Could you check a few things on this model? Use its own coordinates, in mm. Round coordinates to 2 decimals unless told otherwise and drop trailing zeros. Loops run counter-clockwise (first coordinate to the right, second up) from the corner with the lowest first, then second, coordinate; pieces in that order, holes last. Notation, with made-up numbers: (58, -14.5) -> (110, -14.5) arc R36 cw to (110, 23.5) -> close; hole circle Ø3 at (-4, -13.5). An arc over 180 degrees is marked (long way). Write each question's results on one line, items separated by ' | '.
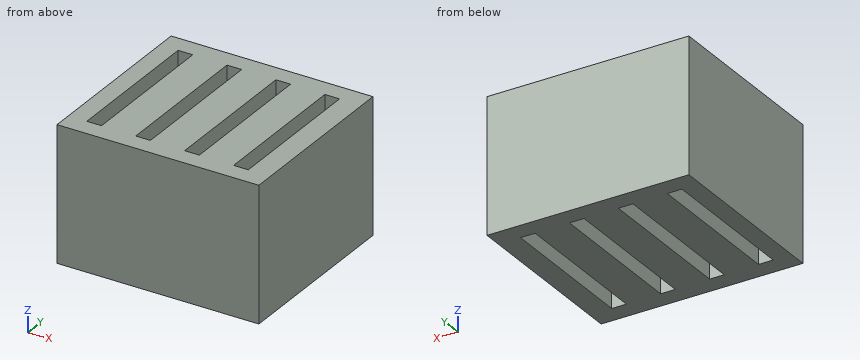
from build123d import *

# Parameters (mm, degrees)
BOX004_W     = 2.4
BOX004_H     = 24
BOX004_DEPTH = 22
BOX002_W     = 2.4
BOX002_H     = 24
BOX002_DEPTH = 22
BOX001_W     = 2.4
BOX001_H     = 24
BOX001_DEPTH = 22
BOX003_W     = 2.4
BOX003_H     = 24
BOX003_DEPTH = 22
BOX_W        = 33
BOX_H        = 30
BOX_DEPTH    = 22


with BuildPart() as cub004:
    # Box004 → Box004 (new body)
    with BuildSketch(Plane(origin=(24, 0, 0), x_dir=(1, 0, 0), z_dir=(0, 0, 1))):
        with Locations((1.2, 12)):
            Rectangle(BOX004_W, BOX004_H)
    extrude(amount=BOX004_DEPTH)


with BuildPart() as cub002:
    # Box002 → Box002 (new body)
    with BuildSketch(Plane(origin=(8, 0, 0), x_dir=(1, 0, 0), z_dir=(0, 0, 1))):
        with Locations((1.2, 12)):
            Rectangle(BOX002_W, BOX002_H)
    extrude(amount=BOX002_DEPTH)


with BuildPart() as fusion:
    # Box001 → Box001 (new body)
    with BuildSketch(Plane.XY):
        with Locations((1.2, 12)):
            Rectangle(BOX001_W, BOX001_H)
    extrude(amount=BOX001_DEPTH)

    # Fusion: union Cub002
    add(cub002.part)


with BuildPart() as fusion001:
    # Box003 → Box003 (new body)
    with BuildSketch(Plane(origin=(16, 0, 0), x_dir=(1, 0, 0), z_dir=(0, 0, 1))):
        with Locations((1.2, 12)):
            Rectangle(BOX003_W, BOX003_H)
    extrude(amount=BOX003_DEPTH)

    # Fusion001: union Cub004, Fusion
    add(cub004.part)
    add(fusion.part)


with BuildPart() as cut:
    # Box → Box (new body)
    with BuildSketch(Plane(origin=(-3, -3, 0), x_dir=(1, 0, 0), z_dir=(0, 0, 1))):
        with Locations((16.5, 15)):
            Rectangle(BOX_W, BOX_H)
    extrude(amount=BOX_DEPTH)

    # Cut: cut Fusion001
    add(fusion001.part, mode=Mode.SUBTRACT)


solid = cut.part
1) I want a section at B-B, the plane y = 20.5. Write out the boundary of the cut face in (x, z).
Model answer:
outline: (-3, 0) -> (0, 0) -> (0, 22) -> (-3, 22) -> close; (2.4, 0) -> (8, 0) -> (8, 22) -> (2.4, 22) -> close; (10.4, 0) -> (16, 0) -> (16, 22) -> (10.4, 22) -> close; (18.4, 0) -> (24, 0) -> (24, 22) -> (18.4, 22) -> close; (26.4, 0) -> (30, 0) -> (30, 22) -> (26.4, 22) -> close
2) I need wall thicknesses on line 1 (X direction, y = 6, z = 16.75); line 2 (Y direction, x = 9, z = 7.5). Which ranges of each line are inside material? Lowest first, please.
Model answer:
line 1: x = -3 to 0, 2.4 to 8, 10.4 to 16, 18.4 to 24, 26.4 to 30 | line 2: y = -3 to 0, 24 to 27
3) I want a section at C-C, the plane z = 6.75. Write out the boundary of the cut face in (x, y), plus the area to 3 significant figures.
Model answer:
outline: (-3, -3) -> (30, -3) -> (30, 27) -> (-3, 27) -> close; hole (0, 0) -> (2.4, 0) -> (2.4, 24) -> (0, 24) -> close; hole (8, 0) -> (10.4, 0) -> (10.4, 24) -> (8, 24) -> close; hole (16, 0) -> (18.4, 0) -> (18.4, 24) -> (16, 24) -> close; hole (24, 0) -> (26.4, 0) -> (26.4, 24) -> (24, 24) -> close | area: 760 mm2
4) I want a section at A-A, the plane x = 16.5. Write out the boundary of the cut face in (y, z).
Model answer:
outline: (-3, 0) -> (0, 0) -> (0, 22) -> (-3, 22) -> close; (24, 0) -> (27, 0) -> (27, 22) -> (24, 22) -> close
